```python
from build123d import *

# Parameters (mm, degrees)
SKETCH1_R                 = 40
BOSS_EXTRUDE1_DEPTH       = 16
SKETCH2_W                 = 41
SKETCH2_H                 = 41
CUT_EXTRUDE1_DEPTH        = 59.787753827
SKETCH13_W                = 61
SKETCH13_H                = 46
BOSS_EXTRUDE4_DEPTH       = 75
SKETCH14_W                = 49
SKETCH14_H                = 67
CUT_EXTRUDE2_DEPTH        = 35
SKETCH15_W                = 49
SKETCH15_H                = 61
CUT_EXTRUDE3_DEPTH        = 5
FILLET1_R                 = 10
FILLET2_R                 = 5
CUT_EXTRUDE5_REACH        = 110.08
SKETCH17_R                = 41
BOSS_EXTRUDE5_DEPTH       = 16
CUT_EXTRUDE4_DEPTH        = 118.224144271
CUT_EXTRUDE4_DEPTH_BACK   = 118.224144271
SKETCH16_R                = 3
F_5_0MM_DOWEL_HOLE1_D     = 5
F_5_0MM_DOWEL_HOLE1_DEPTH = 25
F_5_0MM_DOWEL_HOLE1_TIP   = 1.502151548
CUT_EXTRUDE7_DEPTH        = 123.446927311
CUT_EXTRUDE7_DEPTH_BACK   = 123.446927311
SKETCH22_W                = 41
SKETCH22_H                = 41


with BuildPart() as part:
    # Sketch1 → Boss-Extrude1 (new body)
    with BuildSketch(Plane(origin=(0, 0, 0), x_dir=(1, 0, 0), z_dir=(0, 1, 0))):
        with Locations(Location((0, 0, 0), (0, 0, 270))):
            Circle(SKETCH1_R)
    extrude(amount=BOSS_EXTRUDE1_DEPTH)

    # Sketch2 → Cut-Extrude1 (cut, through all)
    with BuildSketch(Plane(origin=(0, 16, 0), x_dir=(1, 0, 0), z_dir=(0, 1, 0))):
        Rectangle(SKETCH2_W, SKETCH2_H)
    extrude(amount=-CUT_EXTRUDE1_DEPTH, mode=Mode.SUBTRACT)

    # Sketch13 → Boss-Extrude4 (add)
    with BuildSketch(Plane(origin=(0, 0, 20.5), x_dir=(-1, 0, 0), z_dir=(0, 0, -1))):
        with Locations((0, 8)):
            Rectangle(SKETCH13_W, SKETCH13_H)
    extrude(amount=-BOSS_EXTRUDE4_DEPTH)

    # Sketch14 → Cut-Extrude2 (cut)
    with BuildSketch(Plane(origin=(0, 31, 0), x_dir=(1, 0, 0), z_dir=(0, 1, 0))):
        with Locations((0, -62)):
            Rectangle(SKETCH14_W, SKETCH14_H)
    extrude(amount=-CUT_EXTRUDE2_DEPTH, mode=Mode.SUBTRACT)

    # Sketch15 → Cut-Extrude3 (cut)
    with BuildSketch(Plane(origin=(0, -4, 0), x_dir=(1, 0, 0), z_dir=(0, 1, 0))):
        with Locations((0, -59)):
            Rectangle(SKETCH15_W, SKETCH15_H)
    extrude(amount=-CUT_EXTRUDE3_DEPTH, mode=Mode.SUBTRACT)

    # Fillet1
    fillet1_edges = [part.edges().sort_by_distance(p)[0] for p in [
        (-27.5, 31, 95.5),
        (27.5, 31, 95.5),
    ]]
    fillet(fillet1_edges, radius=FILLET1_R)

    # Fillet2
    fillet2_edges = [part.edges().sort_by_distance(p)[0] for p in [
        (0, -9, 89.5),
        (0, -15, 95.5),
        (0, -15, 20.5),
        (0, -9, 28.5),
    ]]
    fillet(fillet2_edges, radius=FILLET2_R - 0.0001)  # a hair under: the kernel refuses the full size

    # Sketch17 → Cut-Extrude5 (cut, up to next)
    with BuildSketch(Plane(origin=(0, 16, 0), x_dir=(1, 0, 0), z_dir=(0, 1, 0)), mode=Mode.PRIVATE) as cut_extrude5_sk1:
        Circle(SKETCH17_R)
    cut_extrude5_tool1 = extrude(cut_extrude5_sk1.sketch, amount=CUT_EXTRUDE5_REACH, mode=Mode.PRIVATE) & part.part
    add(cut_extrude5_tool1.solids().sort_by_distance((0, 16, 0))[0], mode=Mode.SUBTRACT)

    # Sketch18 → Boss-Extrude5 (add)
    with BuildSketch(Plane(origin=(0, 16, 0), x_dir=(1, 0, 0), z_dir=(0, 1, 0))):
        Polygon((20.5, 0), (20.5, -20.5), (-20.5, -20.5), (-20.5, 0), (-40, 0), (-40, -32.874762357), (-24.5, -32.874762357), (-24.5, -28.5), (24.5, -28.5), (24.5, -32.874762357), (40, -32.874762357), (40, 0), align=None)
    extrude(amount=-BOSS_EXTRUDE5_DEPTH)

    # Sketch16 → Cut-Extrude4 (cut, two sides: drawn at the far end of the back side and taken through both)
    with BuildSketch(Plane.ZY.offset(-20.5).offset(-CUT_EXTRUDE4_DEPTH_BACK)):
        with Locations(Location((0, 8, 0), (0, 0, 270))):
            Circle(SKETCH16_R)
    extrude(amount=CUT_EXTRUDE4_DEPTH + CUT_EXTRUDE4_DEPTH_BACK, mode=Mode.SUBTRACT)

    # Ø5.0mm Dowel Hole1
    with Locations(Plane(origin=(-35.25, 8, 32.874762357), x_dir=(1, 0, 0), z_dir=(0, 0, 1))):
        with Locations((0, 0), (70.5, 0)):
            Hole(F_5_0MM_DOWEL_HOLE1_D / 2, depth=F_5_0MM_DOWEL_HOLE1_DEPTH)
            with Locations((0, 0, -(F_5_0MM_DOWEL_HOLE1_DEPTH + F_5_0MM_DOWEL_HOLE1_TIP / 2))):  # 118° drill point
                Cone(0, F_5_0MM_DOWEL_HOLE1_D / 2, F_5_0MM_DOWEL_HOLE1_TIP, mode=Mode.SUBTRACT)

    # Sketch22 → Cut-Extrude7 (cut, two sides: drawn at the far end of the back side and taken through both)
    with BuildSketch(Plane(origin=(0, 16, -16), x_dir=(1, 0, 0), z_dir=(0, -1, 0)).offset(-CUT_EXTRUDE7_DEPTH_BACK)):
        with Locations((0, 16)):
            Rectangle(SKETCH22_W, SKETCH22_H)
        with BuildLine():
            Line((40, 16), (40, 36.5))
            Line((40, 36.5), (20.5, 36.5))
            Line((20.5, 36.5), (20.5, -4.5))
            Line((20.5, -4.5), (-20.5, -4.5))
            Line((-20.5, -4.5), (-20.5, 36.5))
            Line((-20.5, 36.5), (-40, 36.5))
            Line((-40, 36.5), (-40, 16))
            ThreePointArc((-40, 16), (-28.284271226, -12.284271269), (6.1e-08, -24))
            ThreePointArc((6.1e-08, -24), (28.284271269, -12.284271226), (40, 16))
        make_face()
        with BuildLine():
            Line((40, -24), (40, 16))
            ThreePointArc((40, 16), (28.284271269, -12.284271226), (6.1e-08, -24))
            Line((6.1e-08, -24), (40, -24))
        make_face()
        with BuildLine():
            Line((-40, -24), (6.1e-08, -24))
            ThreePointArc((6.1e-08, -24), (-28.284271226, -12.284271269), (-40, 16))
            Line((-40, 16), (-40, -24))
        make_face()
    extrude(amount=CUT_EXTRUDE7_DEPTH + CUT_EXTRUDE7_DEPTH_BACK, mode=Mode.SUBTRACT)


solid = part.part
```
Work out the finished part from the listing and answer in its coordinate system (mm). A direction names the side the tool comes from. Round coordinates to 2 decimals unless told otherwise and drop trailing zeros. Loops run counter-clockwise (first coordinate to the right, second up) from the corner with the lowest first, then second, coordinate; pieces in that order, holes last. Notation, with made-up numbers: M -24,68.25 L -5,68.25 A28 cw -5,103.25 Z; hole C 9,86.5 d5. An arc over 180 degrees is marked long. One line per question, with ' | ' between items.
Q1. Each of these flat-tipped pins is pushed along its axis until it touches: pin 1 Ø7.5 at (x, z) = (36.5, 26.5) entering from -Y; pin 2 Ø24.5 at (x, z) = (-2.5, 57) entering from +Y; pin 3 Ø6 at (x, y) = (11, 10) entering from +Z; pin 4 Ø4 at (x, y) = (35.25, 8) entering from -Z. Where does it stop, or does it pass through?
Conclusion:
pin 1: stops at y = 0 | pin 2: stops at y = -9 | pin 3: stops at z = 28.5 | pin 4: passes through
Q2. The mould has two halves that part along Z. Classify faces 1 (the cylindrical face through (-27.54, 27.99, 92.65)), 2 (the cylindrical face through (0.34, -7.5, 88.07)), 3 (the flat face through (30.5, 8, 57)): +Z half, -Z half, draft (parallel to the pull), parting line (faces both ways), or undercut.
Conclusion:
face 1: +Z half | face 2: undercut | face 3: draft
Q3. A tool of negligible diameter and unlimited length cuts with its end or side. For faces 4 (the flat face through (-35, 0, 27)), 5 (the flat face through (0, -9, 59)), 6 (the flat face through (-33, 6, 32.875)), 7 (the flat face through (37, 6, 32.875)), 8 (the flat face through (0, 6, 28.5)), from which of +Z, -Z, +X, -X, +Y, -Y can it reach the whole face along a straight path? Write none if from no direction.
Conclusion:
face 4: +Z, -Z, -X, -Y | face 5: +Y | face 6: +Z, -X, +Y, -Y | face 7: +Z, +X, +Y, -Y | face 8: +Z, +Y
Q4. Find section A-A, the plane x = 35.25. Give the vertices of the cut face in (y, z).
Conclusion:
outline: M 0,20.5 L 5.5,20.5 L 5.5,32.87 L 0,32.87 Z; M 10.5,20.5 L 16,20.5 L 16,32.87 L 10.5,32.87 Z
Q5. Find section B-B, the plane y = 8. Give the vertices of the cut face in (x, z).
Conclusion:
outline: M -40,20.5 L -37.75,20.5 L -37.75,32.87 L -40,32.87 Z; M -32.75,20.5 L 32.75,20.5 L 32.75,32.87 L 30.5,32.87 L 30.5,95.5 L 24.5,95.5 L 24.5,28.5 L -24.5,28.5 L -24.5,95.5 L -30.5,95.5 L -30.5,32.87 L -32.75,32.87 Z; M 37.75,20.5 L 40,20.5 L 40,32.87 L 37.75,32.87 Z
Q6. Consider line 1 along Y through (x, z) = (35, 27); line 2 along X through (y, z) = (12.5, 50); line 3 along Y through (x, z) = (31, 25.5). Determine where each line is inside the solid, lowest interval first. Write a range as from..to.
Conclusion:
line 1: y = 0..5.51, 10.49..16 | line 2: x = -30.5..-24.5, 24.5..30.5 | line 3: y = 0..16
Q7. Find section C-C, the plane y = 27. Give the vertices of the cut face in (x, z).
Conclusion:
outline: M -30.5,27.4 A41 cw -24.5,32.87 L -24.5,93.5 L -30.5,93.5 Z; M 24.5,32.87 A41 cw 30.5,27.4 L 30.5,93.5 L 24.5,93.5 Z
